Here's the drawing with two shaded views (mm, measured from the low corner). I have some questions. A direction names the side the tool comes from. Give positions to 0.01 mm unless a question says otherwise; leave off trailing zeros. Write each loop counter-clockwise with the first axis right and the second up, starting at its lowest first coordinate (ties: lowest second). Pieces come first, ordered by that corner, then holes. Notation, with made-up numbers: (48.25, 6) -> (102.25, 6) arc R20 cw to (102.25, 30) -> close; hole circle Ø3 at (-24.5, -11). An arc over 180 degrees is marked (long way). One line per item, written item: value.
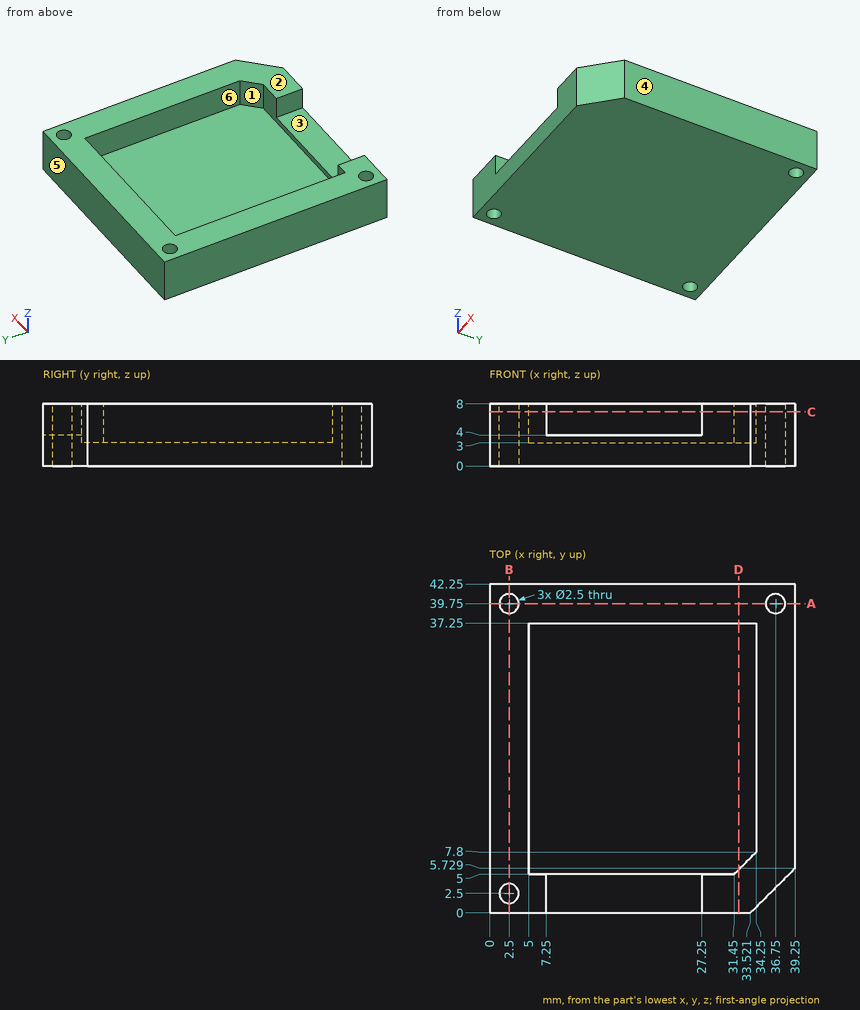
1) If we section it at B-B (x = 2.5): Write out the boundary of the cut face in (y, z).
Answer list:
outline: (0, 0) -> (1.25, 0) -> (1.25, 8) -> (0, 8) -> close; (3.75, 0) -> (38.5, 0) -> (38.5, 8) -> (3.75, 8) -> close; (41, 0) -> (42.25, 0) -> (42.25, 8) -> (41, 8) -> close
2) If we section it at D-D (x = 32): Write out the boundary of the cut face in (y, z).
Answer list:
outline: (0, 0) -> (42.25, 0) -> (42.25, 8) -> (37.25, 8) -> (37.25, 3) -> (5.55, 3) -> (5.55, 8) -> (0, 8) -> close
3) We'd pull the mould along X, two halves only. Please class the marked faces 4, 5 and 6: released by +X, released by -X, zero draft, split by the parting line, or undercut.
Answer list:
face 4: released by +X
face 5: zero draft
face 6: undercut
4) Will these pins go through, and if not, where does the flat tip stop? pin 1 (4 mm diameter, centred on x = 13.5, y = 16, fed in from +Z); pin 2 (1.5 mm diameter, centred on x = 19.5, y = 2, fed in from +Z); pin 3 (3 mm diameter, centred on y = 10.5, z = 3.5, fed in from -X); pin 4 (2 mm diameter, centred on y = 2.5, z = 6, fed in from +X).
Answer list:
pin 1: stops at z = 3
pin 2: stops at z = 4
pin 3: stops at x = 0
pin 4: stops at x = 37.02
5) For the marked faces 1, 2 and 3, which set-ups out of +Z, -Z, +X, -X, +Y, -Y let a thin tool reach every point of the face, with its end or its side?
Answer list:
face 1: +Z
face 2: +Z, +X, -X, +Y, -Y
face 3: +Z, -Y
6) I need wall thicknesses on L1, parallel to Y at x = 2.5, z = 3.25; L2, parallel to Y at x = 6.5, z = 7.5; L3, parallel to X at y = 33, z = 5.75. Which ranges of each line are inside material? Lowest first, please.
Answer list:
L1: y = 0 to 1.25, 3.75 to 38.5, 41 to 42.25
L2: y = 0 to 5, 37.25 to 42.25
L3: x = 0 to 5, 34.25 to 39.25
7) If we section it at A-A (y = 39.75): Write out the boundary of the cut face in (x, z), and give its area (3 significant figures).
Answer list:
outline: (0, 0) -> (1.25, 0) -> (1.25, 8) -> (0, 8) -> close; (3.75, 0) -> (35.5, 0) -> (35.5, 8) -> (3.75, 8) -> close; (38, 0) -> (39.25, 0) -> (39.25, 8) -> (38, 8) -> close
area: 274 mm^2
8) If we section it at C-C (z = 7): Write out the boundary of the cut face in (x, y).
Answer list:
outline: (0, 0) -> (7.25, 0) -> (7.25, 5) -> (5, 5) -> (5, 37.25) -> (34.25, 37.25) -> (34.25, 7.8) -> (31.45, 5) -> (27.25, 5) -> (27.25, 0) -> (33.52, 0) -> (39.25, 5.73) -> (39.25, 42.25) -> (0, 42.25) -> close; hole circle Ø2.5 at (2.5, 2.5); hole circle Ø2.5 at (2.5, 39.75); hole circle Ø2.5 at (36.75, 39.75)
